```python
from build123d import *

# Parameters (mm, degrees)
F0_W     = 140
F0_H     = 140
F1_DEPTH = 140
F2_W     = 130
F2_H     = 130
F3_DEPTH = 60
F4_W     = 130
F4_H     = 70
F5_DEPTH = 130


with BuildPart() as f1:
    # F0 (on Top) → F1 (new body)
    with BuildSketch(Plane.XY):
        Rectangle(F0_W, F0_H)
    extrude(amount=F1_DEPTH)

    # F2 (on face) → F3 (cut)
    with BuildSketch(Plane.XY.offset(140)):
        Rectangle(F2_W, F2_H)
    extrude(amount=-F3_DEPTH, mode=Mode.SUBTRACT)

    # F4 (on face) → F5 (cut)
    with BuildSketch(Plane.XZ.offset(70)):
        with Locations((-0.203013, 40.872386)):
            Rectangle(F4_W, F4_H)
    extrude(amount=-F5_DEPTH, mode=Mode.SUBTRACT)


solid = f1.part
```
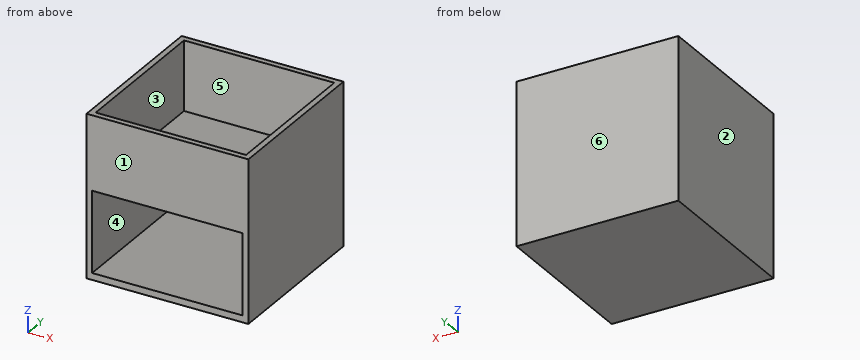
CAD build for the part. Positions are in the model's coordinates, mm. Face numbers are marked on the shaded views. A direction names the side the tool comes from. Round coordinates to 2 decimals unless told otherwise and drop trailing zeros. Loops run counter-clockwise (first coordinate to the right, second up) from the corner with the lowest first, then second, coordinate; pieces in that order, holes last. Notation, with made-up numbers: M -27.5,14 L 5.5,14 A27 cw 5.5,52 Z; hole C 43,75 d2. An arc over 180 degrees is marked long. Use a Markdown table: item, result. Add a question column.
(1) Pull direction Y, two halves, no side cores. Call the marked faces 1, 2 and 3: +Y half, -Y half, draft (parallel to the pull), parting line (faces both ways), or undercut.
(2) Which spindle directions (+Z, -Z, +X, -X, +Y, -Y) get a long thin tool onto all of the face, cutting with end or side? Do the marked faces 4, 5 and 6. Say none if no direction does.
(3) Cut at C-C (z = 110). Give the cut face in (x, y), and give its area (3 significant figures).
(4) Flat gauge pins, fed straight in: pin 1 (21 mm diameter, centred on x = 21.5, z = 29, fed in from -Y); pin 2 (6 mm diameter, centred on x = 52, y = 41.5, fed in from -Z); pin 3 (8 mm diameter, centred on x = -48, y = -25.5, fed in from +Z). Where does each tip first touch, or does it go through?
(5) Drill centre lines: line 1 (X direction, y = -34, z = 34); line 2 (Z direction, x = 28, y = -12.5); line 3 (Y direction, x = 60, z = 124). Where is each one in solid material? Low to high.
(6) Cut at B-B (x = -19.5). Give the cut face in (y, z).
(7) Cut at D-D (z = 13.5). Give the cut face in (x, y), and give its area (3 significant figures).
(8) Cut at A-A (y = -47). Give the cut face in (x, z).
Geometry says:
| question | item | result |
|---|---|---|
| 1 | face 1 | -Y half |
| 1 | face 2 | draft |
| 1 | face 3 | undercut |
| 2 | face 4 | -Y |
| 2 | face 5 | +Z |
| 2 | face 6 | +Z, -Z, +X, -X, +Y |
| 3 | outline | M -70,-70 L 70,-70 L 70,70 L -70,70 Z; hole M -65,-65 L 65,-65 L 65,65 L -65,65 Z |
| 3 | area | 2,700 mm² |
| 4 | pin 1 | stops at y = 60 |
| 4 | pin 2 | stops at z = 0 |
| 4 | pin 3 | stops at z = 80 |
| 5 | line 1 | x = -70 to -65.2, 64.8 to 70 |
| 5 | line 2 | z = 0 to 5.87, 75.87 to 80 |
| 5 | line 3 | y = -70 to -65, 65 to 70 |
| 6 | outline | M -70,0 L 70,0 L 70,140 L 65,140 L 65,80 L -65,80 L -65,140 L -70,140 L -70,75.87 L 60,75.87 L 60,5.87 L -70,5.87 Z |
| 7 | outline | M -70,-70 L -65.2,-70 L -65.2,60 L 64.8,60 L 64.8,-70 L 70,-70 L 70,70 L -70,70 Z |
| 7 | area | 2,700 mm² |
| 8 | outline | M -70,0 L 70,0 L 70,140 L 65,140 L 65,80 L -65,80 L -65,140 L -70,140 Z; hole M -65.2,5.87 L 64.8,5.87 L 64.8,75.87 L -65.2,75.87 Z |
